Study the drawing (mm; zero at the part's minimum x, y, z) and answer. A direction names the side the tool comes from. Round coordinates to 2 decimals unless told otherwise and drop trailing zeros. Order: outer loops, then holes, each group sorted by start corner. A loop starts at its lowest first (then second) coordinate and runs counter-clockwise, first axis right, second up. Notation, with made-up numbers: (19, 62) - (37, 62) arc R28 cw to (37, 80) - close; hole circle Ø8 at (22, 79.25). An arc over 180 degrees is marked (long way). Put each result on its own line as item: value.
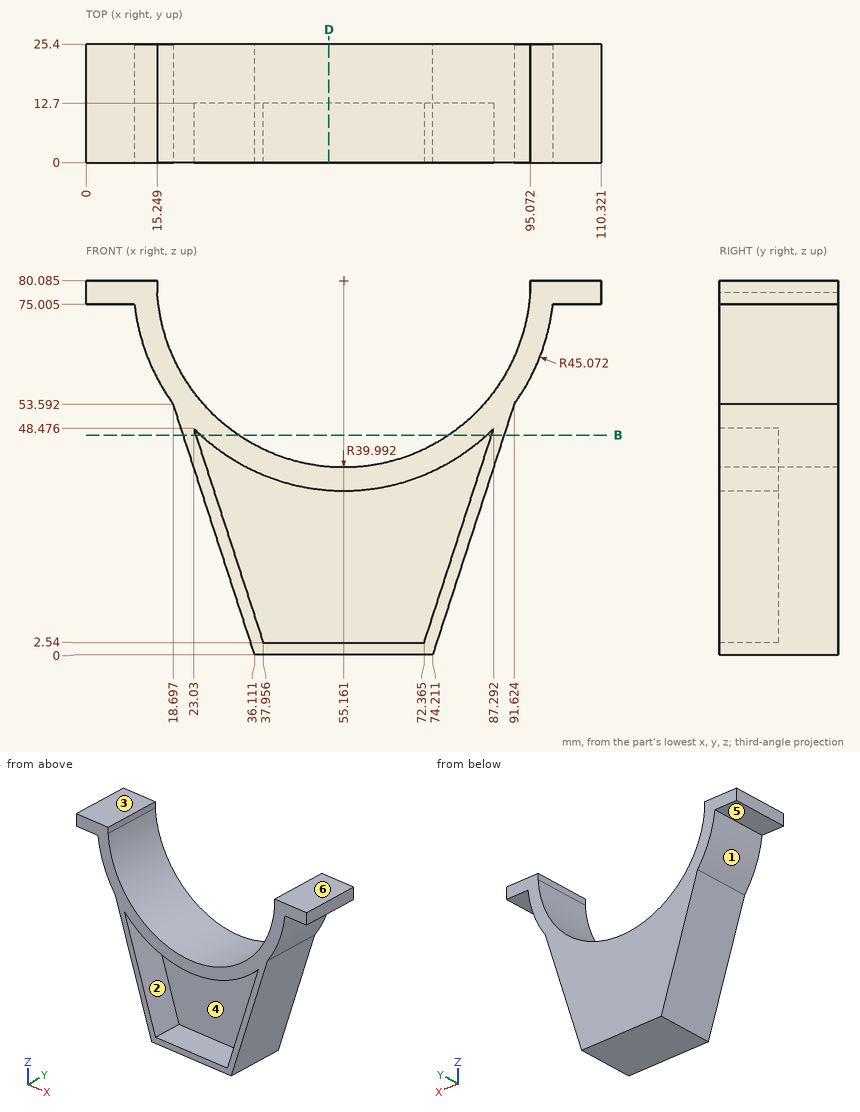
1) A cutting plane is placed at B-B on z = 47. Write down the section's boundary in (x, y) (1 decimal), then the cut area to 3 significant figures.
Findings below:
outline: (20.8, 0) - (23.5, 0) - (23.5, 12.7) - (24.6, 12.7) - (24.6, 0) - (32.7, 0) - (32.7, 25.4) - (20.8, 25.4) - close; (77.6, 0) - (85.8, 0) - (85.8, 12.7) - (86.8, 12.7) - (86.8, 0) - (89.5, 0) - (89.5, 25.4) - (77.6, 25.4) - close
area: 576 mm2
2) Given pin 1 Ø10 at (x, y) = (52.5, 4.5) entering from +Z; pin 2 Ø1 at (x, z) = (13, 65.5) entering from -Y; pin 3 Ø3 at (y, z) = (23, 14.5) entering from -X; pin 4 Ø11.5 at (x, y) = (4.5, 11.5) entering from -Z (1 decimal), each flat-ended and moving along its own axis, determine where each tip first touches the part or whether it passes through.
Findings below:
pin 1: stops at z = 40.83
pin 2: stops at y = 0
pin 3: stops at x = 30.91
pin 4: stops at z = 75
3) A cutting plane is placed at D-D on x = 52. Write down the section's boundary in (y, z).
Findings below:
outline: (0, 0) - (25.4, 0) - (25.4, 40.22) - (0, 40.22) - (0, 35.12) - (12.7, 35.12) - (12.7, 2.54) - (0, 2.54) - close
4) For the marked faces 4, 5 and 6, determine the directions among +Z, -Z, +X, -X, +Y, -Y from which every point of the face is accessible in a straight line to the end or side of a thin tool.
Findings below:
face 4: -Y
face 5: -Z, -X, +Y, -Y
face 6: +Z, +X, -X, +Y, -Y
5) Straight lines are drawn through the part: L1, parallel to Y at x = 48, z = 31.5; L2, parallel to X at y = 6, z = 25 (1 decimal); L3, parallel to Z at x = 101.5, y = 13 (1 decimal). For each, find the intervals that lie inside material, in ascending order. Write a range as from..to.
Findings below:
L1: y = 12.7..25.4
L2: x = 28..30.7, 79.7..82.3
L3: z = 75..80.1
6) For a pull along X with two mould halves and no side action, classify the marked faces 1, 2 and 3 as pulls with the +X half, pulls with the -X half, needs draft (parallel to the pull), parting line crosses it, or undercut.
Findings below:
face 1: pulls with the -X half
face 2: undercut
face 3: needs draft
